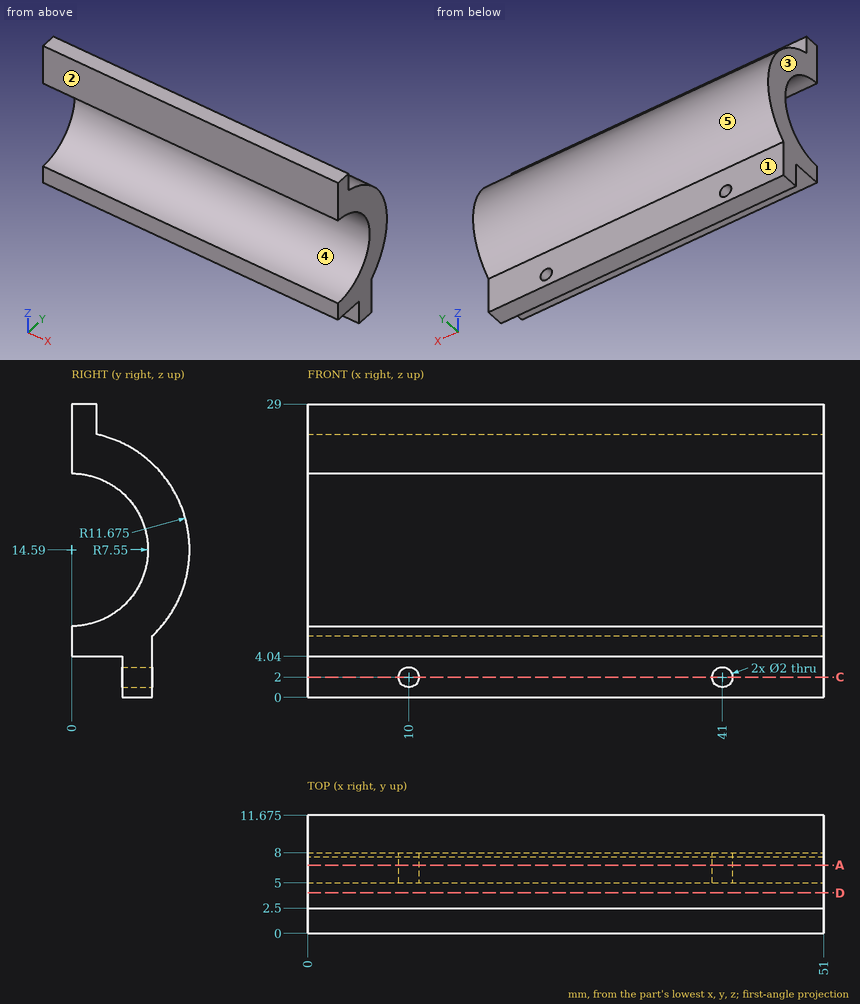
For this review, use the dimensioned drawing (mm, ordinates from the lowest corner) and the shaded views. A direction names the side the tool comes from. Coordinates: 2 decimals unless noted, no trailing zeros. Order: outer loops, then holes, each group sorted by start corner. A loop starts at its lowest first (then second) coordinate and runs counter-clockwise, first axis right, second up. Notation, with made-up numbers: (52, 6.5) -> (63, 6.5) arc R36 ccw to (63, 42.5) -> close; hole circle Ø6 at (63, 72.5). An arc over 180 degrees is marked (long way). One line per item, written item: value. Start each with the question number.
Q1. Tool access review of the marked faces 1 and 2: name each direction out of +Z, -Z, +X, -X, +Y, -Y from which nothing blocks a thin tool from reaching the whole face with its end or side.
Q2. Take a section at C-C, the plane z = 2. State the section outline as (x, y) points.
Q3. For probe 1 along X at (y, z) = (5.8, 2); probe 2 along Z at (x, y) = (41, 6.8); probe 3 along Z at (x, y) = (10, 6.55) (1 decimal), list the stretches that pass through material, from the lowest coordinate up.
Q4. Take a section at A-A, the plane y = 6.75. State the section outline as (x, z) points.
Q5. Insertion check: pin 1 Ø2 at (x, z) = (15, 1.5) entering from -Y; pin 2 Ø1 at (x, z) = (17, 18) entering from -Y; pin 3 Ø0.9 at (x, z) = (25.5, 28) entering from +Y. Each pin has a flat end and moves straight along its axis. Give the tip position at first contact, or say it passes through.
Q6. Take a section at D-D, the plane y = 4. State the section outline as (x, z) points, then the cut area to 3 significant figures.
Q7. Mouldability with a two-part tool opening along Z and no side actions: class the marked faces 3, 4 and 5 as pulls with the +Z half, pulls with the -Z half, needs draft (parallel to the pull), parting line crosses it, or undercut.
Values follow:
1. face 1: -Z, +X, -X, +Y
1. face 2: +Z, -Z, +X, -X, -Y
2. outline: (0, 5) -> (9, 5) -> (9, 8) -> (0, 8) -> close; (11, 5) -> (40, 5) -> (40, 8) -> (11, 8) -> close; (42, 5) -> (51, 5) -> (51, 8) -> (42, 8) -> close
3. probe 1: x = 0 to 9, 11 to 40, 42 to 51
3. probe 2: z = 0 to 1, 3 to 11.31, 17.87 to 24.08
3. probe 3: z = 0 to 1, 3 to 10.8, 18.3 to 24.3
4. outline: (0, 0) -> (51, 0) -> (51, 11.21) -> (0, 11.21) -> close; (0, 17.97) -> (51, 17.97) -> (51, 24.12) -> (0, 24.12) -> close; hole circle Ø2 at (10, 2); hole circle Ø2 at (41, 2)
5. pin 1: stops at y = 5
5. pin 2: stops at y = 6.46
5. pin 3: stops at y = 2.5
6. outline: (0, 4.04) -> (51, 4.04) -> (51, 8.19) -> (0, 8.19) -> close; (0, 20.99) -> (51, 20.99) -> (51, 25.56) -> (0, 25.56) -> close
6. area: 444 mm2
7. face 3: needs draft
7. face 4: undercut
7. face 5: parting line crosses it
